Source: CAD feature listing. Evaluate the final solid. Frame: model axes, mm. Round coordinates to 2 decimals unless told otherwise and drop trailing zeros. Order: outer loops, then holes, each group sorted by start corner. A loop starts at its lowest first (then second) coordinate and runs counter-clockwise, first axis right, second up. Notation, with made-up numbers: (-7, 18.25) - (6, 18.25) arc R11 ccw to (6, 31.25) - close; hole circle Ø10 at (6.5, -38). An arc over 180 degrees is marked (long way). Put each result on its own line as item: value. Start each with the question number.
1) Contact query for flat-ended pins moving along their axis: P1, Ø1.5, axis at x = 33.5, y = -22, coming from the -Z side; P2, Ø12, axis at x = 8, y = -32.5, coming from the +Z side. Output: stop coordinate, or through.
2) Section A-A on y = -21. Output: boundary loops of the cut face in (x, z), then the cut area to 3 significant figures.
3) Section B-B on z = 426. Output: boundary loops of the cut face in (x, y).
4) Line query: probe 1 along X at (y, z) = (-32, 163.5); probe 2 along Y at (x, z) = (13, 1064.5); probe 3 along Y at (x, z) = (4.5, 780.5). Output: solid intervals per line, ascending. Write a range as [from, to].
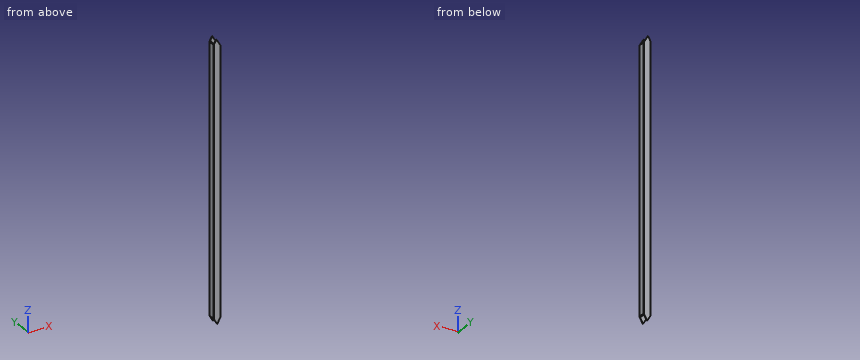
```python
from build123d import *

# Parameters (mm, degrees)
BOSS_EXTRUDE1_DEPTH     = 1500
CUT_EXTRUDE1_DEPTH      = 1501.967428028
CUT_EXTRUDE1_DEPTH_BACK = 1501.967428028
CUT_EXTRUDE2_DEPTH      = 1501.967428028
CUT_EXTRUDE2_DEPTH_BACK = 1501.967428028


with BuildPart() as part:
    # Sketch1 → Boss-Extrude1 (new body)
    with BuildSketch(Plane.XY):
        with BuildLine():
            Line((2.54, 0), (35.56, 0))
            ThreePointArc((35.56, 0), (37.356051224, -0.743948776), (38.1, -2.54))
            Line((38.1, -2.54), (38.1, -35.56))
            ThreePointArc((38.1, -35.56), (37.356051224, -37.356051224), (35.56, -38.1))
            Line((35.56, -38.1), (2.54, -38.1))
            ThreePointArc((2.54, -38.1), (0.743948776, -37.356051224), (0, -35.56))
            Line((0, -35.56), (0, -2.54))
            ThreePointArc((0, -2.54), (0.743948776, -0.743948776), (2.54, 0))
        make_face()
        with BuildLine():
            Line((5.3086, -2.7686), (32.7914, -2.7686))
            ThreePointArc((32.7914, -2.7686), (34.587451224, -3.512548776), (35.3314, -5.3086))
            Line((35.3314, -5.3086), (35.3314, -32.7914))
            ThreePointArc((35.3314, -32.7914), (34.587451224, -34.587451224), (32.7914, -35.3314))
            Line((32.7914, -35.3314), (5.3086, -35.3314))
            ThreePointArc((5.3086, -35.3314), (3.512548776, -34.587451224), (2.7686, -32.7914))
            Line((2.7686, -32.7914), (2.7686, -5.3086))
            ThreePointArc((2.7686, -5.3086), (3.512548776, -3.512548776), (5.3086, -2.7686))
        make_face(mode=Mode.SUBTRACT)
    extrude(amount=BOSS_EXTRUDE1_DEPTH)

    # Sketch2 → Cut-Extrude1 (cut, two sides: drawn at the far end of the back side and taken through both)
    with BuildSketch(Plane(origin=(0, 0, 0), x_dir=(1, 0, 0), z_dir=(0, 1, 0)).offset(-CUT_EXTRUDE1_DEPTH_BACK)):
        Polygon((19.05, 0), (38.1, -32.995567884), (38.1, 0), align=None)
        Polygon((0, -1500), (0, -1474.287456108), (14.845144137, -1500), align=None)
    extrude(amount=CUT_EXTRUDE1_DEPTH + CUT_EXTRUDE1_DEPTH_BACK, mode=Mode.SUBTRACT)

    # Sketch3 → Cut-Extrude2 (cut, two sides: drawn at the far end of the back side and taken through both)
    with BuildSketch(Plane.XZ.offset(38.1).offset(-CUT_EXTRUDE2_DEPTH_BACK)):
        Polygon((35.56, 1500), (14.845144137, 1500), (35.56, 1464.120817175), align=None)
        Polygon((35.56, 1500), (35.56, 1464.120817175), (38.1, 1459.721408123), (38.1, 1500), align=None)
        Polygon((2.54, 0), (2.54, 28.596158833), (0, 32.995567884), (0, 0), align=None)
        Polygon((19.05, 0), (2.54, 28.596158833), (2.54, 0), align=None)
    extrude(amount=CUT_EXTRUDE2_DEPTH + CUT_EXTRUDE2_DEPTH_BACK, mode=Mode.SUBTRACT)


solid = part.part
```
Answer sheet:
1. P1: through
1. P2: z = 1497.31
2. outline: (0, 33) - (2.77, 28.2) - (2.77, 1479.08) - (0, 1474.29) - close; (35.33, 28.2) - (38.1, 33) - (38.1, 1459.72) - (35.33, 1464.52) - close
2. area: 7,970 mm^2
3. outline: (0, -35.56) arc R2.54 ccw to (2.54, -38.1) - (35.56, -38.1) arc R2.54 ccw to (38.1, -35.56) - (38.1, -2.54) arc R2.54 ccw to (35.56, 0) - (2.54, 0) arc R2.54 ccw to (0, -2.54) - close; hole (2.77, -32.79) arc R2.54 ccw to (5.31, -35.33) - (32.79, -35.33) arc R2.54 ccw to (35.33, -32.79) - (35.33, -5.31) arc R2.54 ccw to (32.79, -2.77) - (5.31, -2.77) arc R2.54 ccw to (2.77, -5.31) - close
4. probe 1: [0, 2.77], [35.33, 38.1]
4. probe 2: [-38.1, -35.33], [-2.77, 0]
4. probe 3: [-38.1, -35.2], [-2.9, 0]
